from build123d import *

# Parameters (mm, degrees)
F1_DEPTH = 4
F2_R     = 1.35
F3_DEPTH = 1.7
F4_R     = 1.15
F5_DEPTH = 4


with BuildPart() as f1:
    # F0 (on Top) → F1 (new body)
    with BuildSketch(Plane.XY):
        with BuildLine():
            ThreePointArc((0, 4), (-2, 2), (0, 0))
            Line((0, 0), (0, 4))
        make_face()
        with BuildLine():
            Line((0, 4), (0, 0))
            ThreePointArc((0, 0), (1.414214, 0.585786), (2, 2))
            ThreePointArc((2, 2), (1.414214, 3.414214), (0, 4))
        make_face()
        with BuildLine():
            ThreePointArc((2, 2), (1.414214, 0.585786), (0, 0))
            Line((0, 0), (6, 0))
            Line((6, 0), (6, 4))
            Line((6, 4), (0, 4))
            ThreePointArc((0, 4), (1.414214, 3.414214), (2, 2))
        make_face()
    extrude(amount=F1_DEPTH)

    # F2 (on face) → F3 (cut)
    with BuildSketch(Plane.XY.offset(4)):
        with Locations((0, 2)):
            Circle(F2_R)
    extrude(amount=-F3_DEPTH, mode=Mode.SUBTRACT)

    # F4 (on face) → F5 (cut)
    with BuildSketch(Plane.XY.offset(2.3)):
        with Locations((0, 2)):
            Circle(F4_R)
    extrude(amount=-F5_DEPTH, mode=Mode.SUBTRACT)


solid = f1.part
The model under review builds one solid part; all positions refer to its coordinate system, in mm. A direction names the side the tool comes from. Give positions to 0.01 mm unless a question says otherwise; leave off trailing zeros. Loops run counter-clockwise (first coordinate to the right, second up) from the corner with the lowest first, then second, coordinate; pieces in that order, holes last. Notation, with made-up numbers: (77, 21.5) -> (82, 21.5) arc R26 ccw to (82, 38.5) -> close; hole circle Ø11 at (-27.5, 46.25). An arc over 180 degrees is marked (long way). Answer as a JSON object with one key per item and string values. Group by question number.
Q1. Wall thickness on line 1 along X through (y, z) = (1.4, 1.7); line 2 along Y through (x, z) = (-1, 0.2); line 3 along X through (y, z) = (2.8, 2.65): over which ranges is each line inside the solid? List them lowest first.
Q2. Insertion check: pin 1 (1.4 mm diameter, centred on x = 0, y = 1.5, fed in from +Z). The pin has a flat end and moves straight along its axis. Give the tip position at first contact, or say it passes through.
Q3. Draft analysis for pull direction X (two halves, no side actions). For faces 1 (the cylindrical face through (-0.249, 0.877, 1.166)), 2 (the flat face through (6, 2, 2)), 3 (the flat face through (3, 4, 2)), state which applies: pulls with the +X half, pulls with the -X half, needs draft (parallel to the pull), parting line crosses it, or undercut.
Q4. Take a section at A-A (z = 0.6). Write out the cut boundary in (x, y).
Q5. Take a section at B-B (y = 2). Write out the cut boundary in (x, z), plus the area to 3 significant figures.
Q6. Take a section at C-C (x = 1.25). Write out the cut boundary in (y, z).
Q7. Tool access review of faces 4 (the cylindrical face through (-0.29, 0.68, 3.16)), 5 (the flat face through (3, 2, 0)): name each direction out of +Z, -Z, +X, -X, +Y, -Y from which nothing blocks a thin tool from reaching the whole face with its end or side.
Q8. Take a section at D-D (z = 2.45). Write out the cut boundary in (x, y), plus the area to 3 significant figures.
Answer below:
{
 "1": {"line 1": "x = -1.91 to -0.98, 0.98 to 6", "line 2": "y = 0.27 to 1.43, 2.57 to 3.73", "line 3": "x = -1.83 to -1.09, 1.09 to 6"},
 "2": {"pin 1": "stops at z = 2.3"},
 "3": {"face 1": "undercut", "face 2": "pulls with the +X half", "face 3": "needs draft"},
 "4": {"outline": "(0, 0) -> (6, 0) -> (6, 4) -> (0, 4) arc R2 ccw to start; hole circle Ø2.3 at (0, 2)"},
 "5": {"outline": "(-2, 0) -> (-1.15, 0) -> (-1.15, 2.3) -> (-1.35, 2.3) -> (-1.35, 4) -> (-2, 4) -> close; (1.15, 0) -> (6, 0) -> (6, 4) -> (1.35, 4) -> (1.35, 2.3) -> (1.15, 2.3) -> close", "area": "22.1 mm2"},
 "6": {"outline": "(0, 0) -> (4, 0) -> (4, 4) -> (2.51, 4) -> (2.51, 2.3) -> (1.49, 2.3) -> (1.49, 4) -> (0, 4) -> close"},
 "7": {"face 4": "+Z", "face 5": "-Z, +X, -X, +Y, -Y"},
 "8": {"outline": "(0, 0) -> (6, 0) -> (6, 4) -> (0, 4) arc R2 ccw to start; hole circle Ø2.7 at (0, 2)", "area": "24.6 mm2"}
}
